Source: CAD feature listing. Evaluate the final solid. Frame: model axes, mm. A direction names the side the tool comes from. Coordinates: 2 decimals unless noted, no trailing zeros. Write each loop counter-clockwise with the first axis right and the second up, starting at its lowest first coordinate (ties: lowest second). Pieces come first, ordered by that corner, then holes. Notation, with made-up numbers: (-1, -36) - (39, -36) arc R22 cw to (39, 2) - close; hole circle Ø9 at (31.5, -14). An arc over 180 degrees is marked (long way). One line per question, with ' | ' between items. Start each with the question number.
Q1. Cut plane D-D, the plane y = 2.25. Return loops of the section in (x, z).
Q2. Cut plane B-B, the plane z = 10.3. Return loops of the section in (x, y).
Q3. Cut plane C-C, the plane x = -55. Return loops of the section in (y, z).
Q4. Line query: line 1 (X direction, y = 5.5, z = 10.3); line 2 (Z direction, x = -12.5, y = 7.5); line 3 (Z direction, x = 10, y = 6.5). Output: solid intervals per line, ascending.
Q5. Draft query along Z for faces 5 (the face through (27.32, 4.93, 8.09)), 6 (the face through (17.384, 7.535, -20.947)), 7 (the face through (60, 7, -5)). Return one class per face: +Z half, -Z half, draft (parallel to the pull), parting line (faces both ways), or undercut.
Q6. Contact query for flat-ended pins moving along their axis: P1, Ø2.5, axis at y = 2, z = -10, coming from the +X side; P2, Ø2.5, axis at x = 10, y = 8.5, coming from the -Z side; P3, Ø5, axis at x = 43.5, y = 5.5, coming from the +Z side. Output: stop coordinate, or through.
Q7. Cut plane A-A, the plane x = 0. Return loops of the section in (y, z).
Q8. Access query for faces 1 (the face through (-50, 2, -5)), 2 (the face through (45, 6, -15.2)), 3 (the face through (50, 2, -5)), 4 (the face through (-45, 6, -15.2)). Directions: +Z, -Z, +X, -X, +Y, -Y. A direction counts if a zero-diameter tool reaches every point of the face in a straight line with its end or side. Return the directions, or none.
```python
from build123d import *

# Parameters (mm, degrees)
AUFSATZ_LINEAR_AUSTRAGEN1_DEPTH      = 10
SKIZZE6_R                            = 1.9
SKIZZE6_R_2                          = 11.25
SCHNITT_LINEAR_AUSTRAGEN4_DEPTH      = 67.632124385
SKIZZE7_W                            = 20.880821379
SKIZZE7_H                            = 5
SCHNITT_LINEAR_AUSTRAGEN5_DEPTH      = 87.970339772
VERRUNDUNG3_R                        = 15
SCHNITT_LINEAR_AUSTRAGEN6_DEPTH      = 69.73136111
SCHNITT_LINEAR_AUSTRAGEN6_DEPTH_BACK = 69.73136111
SKIZZE8_W                            = 10
SKIZZE8_H                            = 5
SKIZZE9_R                            = 1.7
SCHNITT_LINEAR_AUSTRAGEN7_DEPTH      = 10
AUFSATZ_LINEAR_AUSTRAGEN2_DEPTH      = 5
FASE1_DEPTH                          = 5
VERRUNDUNG6_R                        = 10


with BuildPart() as part:
    # Skizze1 → Aufsatz-Linear austragen1 (new body)
    with BuildSketch(Plane(origin=(0, 0, 0), x_dir=(1, 0, 0), z_dir=(0, 1, 0))):
        Polygon((-60, -4.8), (-22, -4.8), (-22, -16.8), (22, -16.8), (22, -4.8), (60, -4.8), (60, 15.2), (22, 15.2), (22, 27.2), (0, 27.2), (-22, 27.2), (-22, 15.2), (-60, 15.2), align=None)
    extrude(amount=AUFSATZ_LINEAR_AUSTRAGEN1_DEPTH)

    # Skizze6 → Schnitt-Linear austragen4 (cut, through all)
    with BuildSketch(Plane(origin=(0, 10, 0), x_dir=(1, 0, 0), z_dir=(0, 1, 0))):
        with Locations(Location((15.5, 20.7, 0), (0, 0, 270))):
            Circle(SKIZZE6_R)
        with Locations(Location((15.5, -10.3, 0), (0, 0, 270))):
            Circle(SKIZZE6_R)
        with Locations(Location((-15.5, -10.3, 0), (0, 0, 270))):
            Circle(SKIZZE6_R)
        with Locations(Location((-15.5, 20.7, 0), (0, 0, 270))):
            Circle(SKIZZE6_R)
        with Locations(Location((0, 5.2, 0), (0, 0, 270))):
            Circle(SKIZZE6_R_2)
    extrude(amount=-SCHNITT_LINEAR_AUSTRAGEN4_DEPTH, mode=Mode.SUBTRACT)

    # Skizze7 → Schnitt-Linear austragen5 (cut, through all)
    with BuildSketch(Plane.ZY.offset(22)):
        with Locations((-25.64041069, 2.5)):
            Rectangle(SKIZZE7_W, SKIZZE7_H)
    extrude(amount=-SCHNITT_LINEAR_AUSTRAGEN5_DEPTH, mode=Mode.SUBTRACT)

    # Verrundung3
    # the kernel refuses this fillet: 15 mm, written as the material it adds along each edge
    with BuildSketch(Plane(origin=(-22, 5, -15.2), x_dir=(0, 0, -1), z_dir=(0, 1, 0))) as verrundung3_piece_1:
        with BuildLine():
            CenterArc((15, 14.696938457), VERRUNDUNG3_R, 180, 78.463040967)
            Line((0, 14.696938457), (-0.3, 14.696938457))
            Line((-0.3, 14.696938457), (-0.3, 0))
            Line((-0.3, 0), (0, -0.3))
            ThreePointArc((0, -0.3), (6, -0.3), (11.94, -0.293938769))
            Line((11.94, -0.293938769), (12, 0))
        make_face()
    extrude(amount=5)
    with BuildSketch(Plane(origin=(-22, 0, 4.8), x_dir=(-1, 0, 0), z_dir=(0, 1, 0))) as verrundung3_piece_2:
        with BuildLine():
            CenterArc((14.696938457, 15), VERRUNDUNG3_R, 191.536959033, 78.463040967)
            Line((0, 12), (-0.293938769, 11.94))
            ThreePointArc((-0.293938769, 11.94), (-0.3, 6), (-0.3, 0))
            Line((-0.3, 0), (0, -0.3))
            Line((0, -0.3), (14.696938457, -0.3))
            Line((14.696938457, -0.3), (14.696938457, 0))
        make_face()
    extrude(amount=10)
    with BuildSketch(Plane(origin=(22, 0, 4.8), x_dir=(1, 0, 0), z_dir=(0, 1, 0))) as verrundung3_piece_3:
        with BuildLine():
            CenterArc((14.696938457, -15), VERRUNDUNG3_R, 90, 78.463040967)
            Line((0, -12), (-0.293938769, -11.94))
            ThreePointArc((-0.293938769, -11.94), (-0.3, -6), (-0.3, 0))
            Line((-0.3, 0), (0, 0.3))
            Line((0, 0.3), (14.696938457, 0.3))
            Line((14.696938457, 0.3), (14.696938457, 0))
        make_face()
    extrude(amount=10)
    with BuildSketch(Plane(origin=(22, 5, -15.2), x_dir=(1, 0, 0), z_dir=(0, 1, 0))) as verrundung3_piece_4:
        with BuildLine():
            CenterArc((14.696938457, 15), VERRUNDUNG3_R, 191.536959033, 78.463040967)
            Line((0, 12), (-0.293938769, 11.94))
            ThreePointArc((-0.293938769, 11.94), (-0.3, 6), (-0.3, 0))
            Line((-0.3, 0), (0, -0.3))
            Line((0, -0.3), (14.696938457, -0.3))
            Line((14.696938457, -0.3), (14.696938457, 0))
        make_face()
    extrude(amount=5)

    # Skizze8 → Schnitt-Linear austragen6 (cut, two sides: drawn at the far end of the back side and taken through both)
    with BuildSketch(Plane(origin=(0, 0, -15.2), x_dir=(-1, 0, 0), z_dir=(0, 0, -1)).offset(-SCHNITT_LINEAR_AUSTRAGEN6_DEPTH_BACK)):
        with Locations((-55, 2.5)):
            Rectangle(SKIZZE8_W, SKIZZE8_H)
        with Locations((55, 2.5)):
            Rectangle(SKIZZE8_W, SKIZZE8_H)
    extrude(amount=SCHNITT_LINEAR_AUSTRAGEN6_DEPTH + SCHNITT_LINEAR_AUSTRAGEN6_DEPTH_BACK, mode=Mode.SUBTRACT)

    # Skizze9 → Schnitt-Linear austragen7 (cut)
    with BuildSketch(Plane.XZ.offset(-5)):
        with Locations(Location((-55, -0.2, 0), (0, 0, 270))):
            Circle(SKIZZE9_R)
        with Locations(Location((-55, -10.2, 0), (0, 0, 90))):
            Circle(SKIZZE9_R)
        with Locations(Location((55, -10.2, 0), (0, 0, 270))):
            Circle(SKIZZE9_R)
        with Locations(Location((55, -0.2, 0), (0, 0, 90))):
            Circle(SKIZZE9_R)
    extrude(amount=-SCHNITT_LINEAR_AUSTRAGEN7_DEPTH, mode=Mode.SUBTRACT)

    # Skizze10 → Aufsatz-Linear austragen2 (add)
    with BuildSketch(Plane(origin=(0, 10, 0), x_dir=(1, 0, 0), z_dir=(0, 1, 0))):
        Polygon((-22, 27.2), (-20.360366379, 29.068218634), (-18.720732758, 27.2), align=None)
    extrude(amount=-AUFSATZ_LINEAR_AUSTRAGEN2_DEPTH)

    # Fase1: read off the stored shape, not the designer's step
    # Fase1 outline → Fase1 (cut)
    with BuildSketch(Plane(origin=(0, 0, 0), x_dir=(1, 0, 0), z_dir=(0, 1, 0))):
        with BuildLine():
            Line((-5.153882032, 15.2), (-33.153882032, 15.2))
            Line((-33.153882032, 15.2), (-8.71856035, -1.90979644))
            ThreePointArc((-8.71856035, -1.90979644), (-11.013512063, 7.494570119), (-5.153882032, 15.2))
        make_face()
        with BuildLine():
            ThreePointArc((5.153882032, 15.2), (11.013512063, 7.494570119), (8.71856035, -1.90979644))
            Line((8.71856035, -1.90979644), (33.153882032, 15.2))
            Line((33.153882032, 15.2), (5.153882032, 15.2))
        make_face()
    extrude(amount=FASE1_DEPTH, mode=Mode.SUBTRACT)

    # Verrundung6
    verrundung6_edges = [part.edges().sort_by_distance(p)[0] for p in [
        (8.71856035, 2.5, 1.90979644),
        (-8.71856035, 2.5, 1.90979644),
        (-33.153882032, 2.5, -15.2),
        (33.153882032, 2.5, -15.2),
    ]]
    fillet(verrundung6_edges, radius=VERRUNDUNG6_R)


solid = part.part
```
Reply:
1) outline: (-50, -15.2) - (-36.31, -15.2) arc R10 ccw to (-30.57, -13.39) - (-9.67, 1.24) arc R10 ccw to (-8.16, 2.55) arc R11.25 cw to (8.16, 2.55) arc R10 ccw to (9.67, 1.24) - (30.57, -13.39) arc R10 ccw to (36.31, -15.2) - (50, -15.2) - (50, 4.8) - (36.7, 4.8) arc R15 cw to (22, 16.8) - (-22, 16.8) arc R15 cw to (-36.7, 4.8) - (-50, 4.8) - close; hole circle Ø3.8 at (-15.5, 10.3); hole circle Ø3.8 at (15.5, 10.3)
2) outline: (-25.09, 0) - (-17.4, 0) - (-17.4, 10) - (-25.09, 10) - close; (-13.6, 0) - (13.6, 0) - (13.6, 10) - (-13.6, 10) - close; (17.4, 0) - (25.09, 0) - (25.09, 10) - (17.4, 10) - close
3) outline: (5, -15.2) - (10, -15.2) - (10, -11.9) - (5, -11.9) - close; (5, -8.5) - (10, -8.5) - (10, -1.9) - (5, -1.9) - close; (5, 1.5) - (10, 1.5) - (10, 4.8) - (5, 4.8) - close
4) line 1: x = -25.09 to -17.4, -13.6 to 13.6, 17.4 to 25.09 | line 2: z = -27.2 to 16.8 | line 3: z = -27.2 to -10.35, -0.05 to 16.8
5) face 5: +Z half | face 6: undercut | face 7: draft
6) P1: stops at x = 50 | P2: stops at z = -27.2 | P3: stops at z = 4.8
7) outline: (0, 6.05) - (10, 6.05) - (10, 16.8) - (0, 16.8) - close; (5, -27.2) - (10, -27.2) - (10, -16.45) - (5, -16.45) - close
8) face 1: +Z, -Z, -X, -Y | face 2: -Z, +X, +Y, -Y | face 3: +Z, -Z, +X, -Y | face 4: -Z, -X, +Y, -Y
